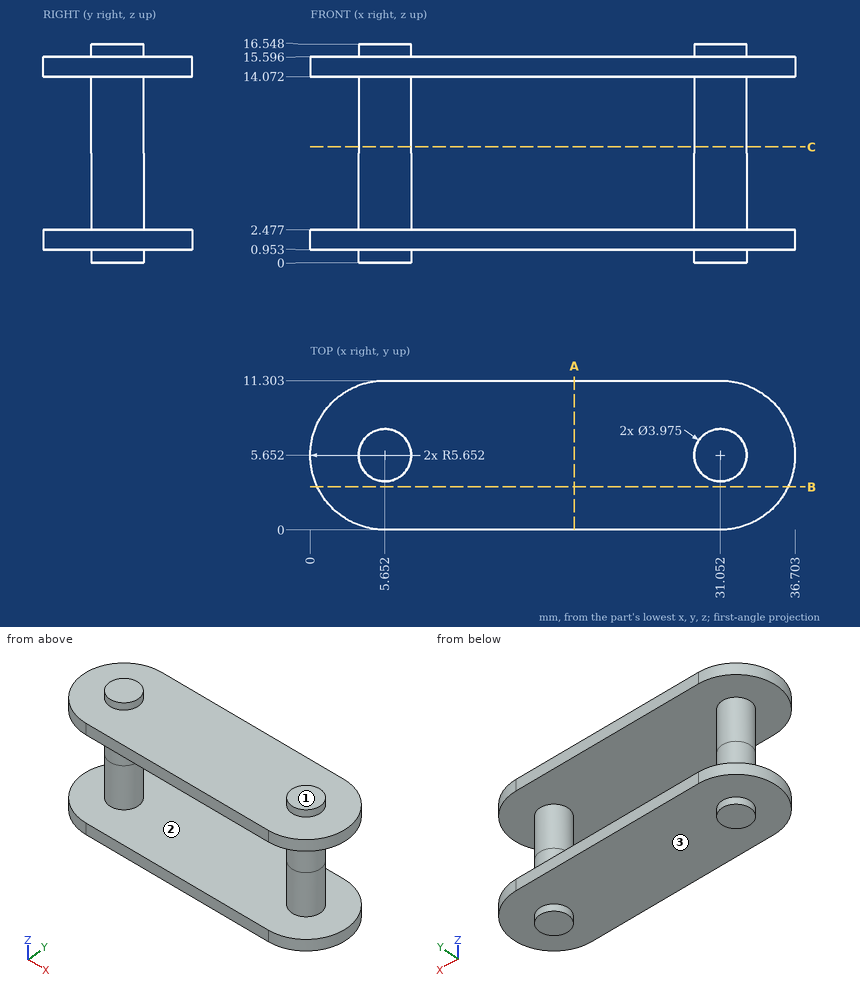
Here's the drawing with two shaded views (mm, measured from the low corner). I have some questions. Round coordinates to 2 decimals unless told otherwise and drop trailing zeros. Order: outer loops, then holes, each group sorted by start corner. A loop starts at its lowest first (then second) coordinate and runs counter-clockwise, first axis right, second up. Notation, with made-up numbers: (-20, 64.5) -> (-16, 64.5) arc R26 ccw to (-16, 89.5) -> close; hole circle Ø11 at (6, 35). An arc over 180 degrees is marked (long way). Use a Markdown table: item, result. Add a question column.
(1) For pin 1 Ø5 at (x, z) = (25.5, 3.5) entering from +Y; pin 2 Ø3.5 at (x, y) = (22, 4.5) entering from +Z; pin 3 Ø5.5 at (x, y) = (19.5, 6.5) entering from -Z, each with a flat end and sliding along its axis, tell me the tip position at first contact or that it passes through.
(2) I need wall thicknesses on line 1 along Z through (x, y) = (33, 1.75) (1 decimal); line 2 along X through (y, z) = (4, 4.5) (1 decimal); line 3 along X through (y, z) = (7, 12). Which ranges of each line are inside material? Lowest first, please.
(3) Suppose I cut it at C-C, the plane z = 8.75. Please give me the cut outline in (x, y) (1 decimal).
(4) Suppose I cut it at A-A, the plane x = 20. Please give me the cut outline in (y, z) (1 decimal).
(5) Suppose I cut it at B-B, the plane y = 3.25. Please give me the cut outline in (x, z) (1 decimal).
(6) If we mould it in two halves opening along Z, with no side actions, what happens to the marked faces 1, 2 and 3? For each: released by +Z, released by -Z, zero draft, split by the parting line, or undercut.
Verdict:
| question | item | result |
|---|---|---|
| 1 | pin 1 | y = 11.3 |
| 1 | pin 2 | z = 15.6 |
| 1 | pin 3 | z = 0.95 |
| 2 | line 1 | 1 to 2.5, 14.1 to 15.6 |
| 2 | line 2 | 4.5 to 6.8, 29.9 to 32.2 |
| 2 | line 3 | 4.19 to 7.11, 29.59 to 32.51 |
| 3 | outline | circle Ø4 at (5.7, 5.7); circle Ø4 at (31.1, 5.7) |
| 4 | outline | (0, 1) -> (11.3, 1) -> (11.3, 2.5) -> (0, 2.5) -> close; (0, 14.1) -> (11.3, 14.1) -> (11.3, 15.6) -> (0, 15.6) -> close |
| 5 | outline | (0.5, 1) -> (36.2, 1) -> (36.2, 2.5) -> (0.5, 2.5) -> close; (0.5, 14.1) -> (36.2, 14.1) -> (36.2, 15.6) -> (0.5, 15.6) -> close |
| 6 | face 1 | released by +Z |
| 6 | face 2 | undercut |
| 6 | face 3 | released by -Z |
